Check sheet for the modelled part. Datum: model origin and axes. Units: mm. A direction names the side the tool comes from. Round coordinates to 2 decimals unless told otherwise and drop trailing zeros. Write each loop counter-clockwise with the first axis right and the second up, starting at its lowest first coordinate (ties: lowest second). Pieces come first, ordered by that corner, then holes. Notation, with made-up numbers: (-25.5, 87) -> (26.5, 87) arc R17 cw to (26.5, 97) -> close; hole circle Ø4 at (81, 58.5). An arc over 180 degrees is marked (long way). Answer as a JSON object with one key per item and string values. Group by question number.
```python
from build123d import *

# Parameters (mm, degrees)
SKETCH_1_R          = 4
EXTRUDE_1_DEPTH     = 2
SKETCH_2_W          = 30
SKETCH_2_H          = 50
EXTRUDE_2_DEPTH     = 2
CUT_EXTRUDE_1_DEPTH = 55


with BuildPart() as part:
    # 草图1 → 凸台-拉伸1 (new body)
    with BuildSketch(Plane.XY):
        Polygon((-27.530821095, -16.070026793), (37.469178905, -16.070026793), (37.469178905, 13.929973207), (22.469178905, 13.929973207), (22.469178905, 113.929973207), (-13.530821095, 113.929973207), (-13.530821095, 13.929973207), (-27.530821095, 13.929973207), align=None)
        with Locations((21.469178905, 3.929973207)):
            Circle(SKETCH_1_R, mode=Mode.SUBTRACT)
        with Locations((-10.530821095, 3.929973207)):
            Circle(SKETCH_1_R, mode=Mode.SUBTRACT)
    extrude(amount=EXTRUDE_1_DEPTH)

    # 草图2 → 凸台-拉伸2 (add)
    with BuildSketch(Plane(origin=(22.469178905, 0, 0), x_dir=(0, 0, -1), z_dir=(1, 0, 0))):
        with Locations((-15, 88.929973207)):
            Rectangle(SKETCH_2_W, SKETCH_2_H)
    extrude_2 = extrude(amount=EXTRUDE_2_DEPTH)

    # 镜向1: 凸台-拉伸2 across plane
    add(extrude_2.mirror(Plane(origin=(4.969178905, 0, 0), x_dir=(0, 0, 1), z_dir=(1, 0, 0))))

    # 草图3 → 切除-拉伸1 (cut)
    with BuildSketch(Plane(origin=(24.469178905, 0, 0), x_dir=(0, 0, -1), z_dir=(1, 0, 0))):
        with BuildLine():
            Line((-14.837360519, 105.36567793), (-14.837360519, 72.494268484))
            ThreePointArc((-14.837360519, 72.494268484), (-9.837360519, 67.494268484), (-4.837360519, 72.494268484))
            Line((-4.837360519, 72.494268484), (-4.837360519, 105.36567793))
            ThreePointArc((-4.837360519, 105.36567793), (-9.837360519, 110.36567793), (-14.837360519, 105.36567793))
        make_face()
    extrude(amount=-CUT_EXTRUDE_1_DEPTH, mode=Mode.SUBTRACT)


solid = part.part
```
(1) Section check B-B on y = 85. Record the cut outline in (x, z).
(2) Scan lines: line 1 along X through (y, z) = (68.5, 27.75); line 2 along Z through (x, y) = (18, 13.5); line 3 along X through (y, z) = (24, 1.5). Record each from-to range of solid material in increasing order.
(3) Section check C-C on x = -8. Record the cut outline in (y, z), then the cut area to 3 significant figures.
(4) Section check A-A on z = 20.25. Record the cut outline in (x, y), then the cut area to 3 significant figures.
(5) Access from +Z, -Z, +X, -X, +Y, -Y to the whole of each face (thin tool, end or side, straight path). Record for faces 4 (the flat face through (-14.531, 89, 19)), 5 (the flat face through (-12.531, 89, 19)), 6 (the flat face through (24.469, 89, 19)), 7 (the cylindrical face through (-13.517, 110.364, 9.727)).
(6) Go/stop test with flat-tipped pins: pin 1 Ø1.6 at (x, z) = (24, 21.5) entering from -Y; pin 2 Ø1.6 at (x, y) = (23.5, 93.5) entering from -Z; pin 3 Ø13 at (x, y) = (21.47, 3.93) entering from +Z; pin 4 Ø2 at (y, z) = (28, 1.5) entering from +X. Record where each tip stops, or that it passes through.
(7) Section check D-D on z = 8.75. Record the cut outline in (x, y).
(8) Release check for a two-part mould opening along Z. For faces 1 (the flat face through (5, 48, 0)), 2 (the cylindrical face through (-6.716, 5.131, 0.986)), 3 (the cylindrical face through (23.483, 67.495, 9.947)) record: pulls with the +Z half, pulls with the -Z half, needs draft (parallel to the pull), parting line crosses it, or undercut.
Data:
{
 "1": {"outline": "(-14.53, 0) -> (24.47, 0) -> (24.47, 4.84) -> (22.47, 4.84) -> (22.47, 2) -> (-12.53, 2) -> (-12.53, 4.84) -> (-14.53, 4.84) -> close; (-14.53, 14.84) -> (-12.53, 14.84) -> (-12.53, 30) -> (-14.53, 30) -> close; (22.47, 14.84) -> (24.47, 14.84) -> (24.47, 30) -> (22.47, 30) -> close"},
 "2": {"line 1": "x = -14.53 to -12.53, 22.47 to 24.47", "line 2": "z = 0 to 2", "line 3": "x = -13.53 to 22.47"},
 "3": {"outline": "(-16.07, 0) -> (0.83, 0) -> (0.83, 2) -> (-16.07, 2) -> close; (7.03, 0) -> (113.93, 0) -> (113.93, 2) -> (7.03, 2) -> close", "area": "248 mm²"},
 "4": {"outline": "(-14.53, 63.93) -> (-12.53, 63.93) -> (-12.53, 113.93) -> (-14.53, 113.93) -> close; (22.47, 63.93) -> (24.47, 63.93) -> (24.47, 113.93) -> (22.47, 113.93) -> close", "area": "200 mm²"},
 "5": {"face 4": "+Z, -Z, -X, +Y", "face 5": "+Z, +Y, -Y", "face 6": "+Z, -Z, +X, +Y", "face 7": "+X, -X"},
 "6": {"pin 1": "stops at y = 63.93", "pin 2": "stops at z = 0", "pin 3": "stops at z = 2", "pin 4": "stops at x = 22.47"},
 "7": {"outline": "(-14.53, 63.93) -> (-12.53, 63.93) -> (-12.53, 67.61) -> (-14.53, 67.61) -> close; (-14.53, 110.25) -> (-12.53, 110.25) -> (-12.53, 113.93) -> (-14.53, 113.93) -> close; (22.47, 63.93) -> (24.47, 63.93) -> (24.47, 67.61) -> (22.47, 67.61) -> close; (22.47, 110.25) -> (24.47, 110.25) -> (24.47, 113.93) -> (22.47, 113.93) -> close"},
 "8": {"face 1": "pulls with the -Z half", "face 2": "needs draft", "face 3": "undercut"}
}
